Model file for the job. Use its own axes, mm. A direction names the side the tool comes from. Round coordinates to 2 decimals unless told otherwise and drop trailing zeros. Order: outer loops, then holes, each group sorted by start corner. A loop starts at its lowest first (then second) coordinate and runs counter-clockwise, first axis right, second up. Notation, with made-up numbers: (7, -22.75) - (32, -22.75) arc R18 ccw to (32, -8.75) - close; hole circle Ø4 at (24, -17). An arc over 180 degrees is marked (long way). Put each result on its own line as item: value. Start each with the question number.
Item 1: Pin check, flat tips, straight feed: pin 1 Ø5.5 at (x, z) = (-9, 14) entering from -Y; pin 2 Ø2 at (y, z) = (-12.5, 2.5) entering from -X. Stop position of each tip, or through.
Item 2: Saw through at C-C on y = -12. List the corners of the cut face in (x, z), plus the area to 3 significant figures.
Item 3: Saw through at A-A on z = 3.75. List the corners of the cut face in (x, y), plus the area to 3 significant figures.
Item 4: Which spindle directions (+Z, -Z, +X, -X, +Y, -Y) get a long thin tool onto all of the face, cutting with end or side? Do faces 1 (the face through (1.173, -9.295, 19.507)), 2 (the face through (-9, -0.435, 10)), 3 (the face through (-19.334, 10, 10)). Say none if no direction does.
Item 5: Saw through at B-B on x = -10. List the corners of the cut face in (y, z), plus the area to 3 significant figures.
Item 6: Probe probe 1 along Y at (x, z) = (-11, 11.25); probe 2 along X at (y, z) = (-8, 7.25); probe 3 along Z at (x, y) = (-13, 0). List the from-to ranges inside material, lowest first.
```python
from build123d import *

# Parameters (mm, degrees)
F1_DEPTH = 20
F2_SIZE  = 1


with BuildPart() as f1:
    # F0 (on Top) → F1 (new body)
    with BuildSketch(Plane.XY):
        Polygon((20.665561, 19.565226), (-19.334439, 19.565226), (-19.334439, -0.434774), (0.665561, -0.434774), (0.665561, -20.434774), (20.665561, -20.434774), align=None)
    extrude(amount=F1_DEPTH)

    # F2
    f2_edges = [f1.edges().sort_by_distance(p)[0] for p in [
        (0.665561, -20.434774, 10),
        (20.665561, -20.434774, 10),
        (10.665561, -20.434774, 0),
        (10.665561, -20.434774, 20),
        (-19.334439, 19.565226, 10),
        (-19.334439, -0.434774, 10),
        (-19.334439, 9.565226, 0),
        (-19.334439, 9.565226, 20),
        (0.665561, 19.565226, 0),
        (-9.334439, -0.434774, 0),
        (0.665561, -10.434774, 0),
        (20.665561, -0.434774, 0),
        (20.665561, 19.565226, 10),
        (20.665561, -0.434774, 20),
        (0.665561, 19.565226, 20),
        (-9.334439, -0.434774, 20),
        (0.665561, -10.434774, 20),
    ]]
    chamfer(f2_edges, length=F2_SIZE)


solid = f1.part
```
Results found:
1. pin 1: stops at y = -0.43
1. pin 2: stops at x = 0.67
2. outline: (0.67, 1) - (1.67, 0) - (19.67, 0) - (20.67, 1) - (20.67, 19) - (19.67, 20) - (1.67, 20) - (0.67, 19) - close
2. area: 398 mm²
3. outline: (-19.33, 0.57) - (-18.33, -0.43) - (0.67, -0.43) - (0.67, -19.43) - (1.67, -20.43) - (19.67, -20.43) - (20.67, -19.43) - (20.67, 18.57) - (19.67, 19.57) - (-18.33, 19.57) - (-19.33, 18.57) - close
3. area: 1,200 mm²
4. face 1: +Z, -X, -Y
4. face 2: +Z, -Z, -X, -Y
4. face 3: +Z, -Z, -X, +Y, -Y
5. outline: (-0.43, 1) - (0.57, 0) - (18.57, 0) - (19.57, 1) - (19.57, 19) - (18.57, 20) - (0.57, 20) - (-0.43, 19) - close
5. area: 398 mm²
6. probe 1: y = -0.43 to 19.57
6. probe 2: x = 0.67 to 20.67
6. probe 3: z = 0.57 to 19.43
